Autodesk Inventor part; units mm, degrees
ref_plane "YZ Plane" through (0, 0, 0) normal (1, 0, 0) x (0, 1, 0)
ref_plane "XZ Plane" through (0, 0, 0) normal (0, 1, 0) x (-1, 0, 0)
ref_plane "XY Plane" through (0, 0, 0) normal (0, 0, 1) x (1, 0, 0)
sketch "Skizze1" plane through (0, 0, 0) normal (1, 0, 0) x (0, 1, 0)
  arc A0 (10, 59.1608) -> (10, -59.1608) centre (0, 0) ccw
  line L0 (10, 59.1608) -> (10, -9.1608)
  line L1 (10, -59.1608) -> (10, -49.1608)
  line L2 (10, -9.1608) -> (0, -9.1608)
  line L3 (0, -9.1608) -> (0, -49.1608)
  line L4 (0, -49.1608) -> (10, -49.1608)
  circle A1 centre (0, 55) radius 3
  circle A2 centre (-32.3282, 44.4959) radius 3
  circle A3 centre (-52.3081, 16.9959) radius 3
  circle A4 centre (-52.3081, -16.9959) radius 3
  circle A5 centre (-32.3282, -44.4959) radius 3
  circle A6 centre (0, -55) radius 3
  circle A7 centre (0, 0) radius 1.25
  line L5 (-7, 0) -> (-49.1993, 12.5)
  line L6 (-49.1993, 12.5) -> (-49.1993, -12.5)
  line L7 (-49.1993, -12.5) -> (-7, 0)
  line L8 (-74, 0) -> (24, 0)
  line L9 (-33.132, -38.459) -> (-5.7341, -4.015)
  line L10 (-5.7341, -4.015) -> (-47.4714, -17.9802)
  line L11 (-47.4714, -17.9802) -> (-33.132, -38.459)
  line L12 (-5.081, -50.5075) -> (-2.3941, -6.5778)
  line L13 (-2.3941, -6.5778) -> (-28.5733, -41.957)
  line L14 (-28.5733, -41.957) -> (-5.081, -50.5075)
  line L15 (-33.132, 38.459) -> (-5.7341, 4.015)
  line L16 (-5.7341, 4.015) -> (-47.4714, 17.9802)
  line L17 (-47.4714, 17.9802) -> (-33.132, 38.459)
  line L18 (-5.081, 50.5075) -> (-2.3941, 6.5778)
  line L19 (-2.3941, 6.5778) -> (-28.5733, 41.957)
  line L20 (-28.5733, 41.957) -> (-5.081, 50.5075)
  dimension "d0" = 120
  dimension "d1" = 40
  dimension "d2" = 10
  dimension "d3" = 10
  dimension "d4" = 10
  dimension "d5" = 10
  dimension "d6" = 55
  dimension "d7" = 0
  dimension "d8" = 6
  dimension "d11" = 180
  dimension "d13" = 2.5
  dimension "d19" = 33
  dimension "d20" = 12.5
  dimension "d22" = 0
  dimension "d23" = 7
  dimension "d26" = 70
  dimension "d34" = 25
extrude "Extrusion1" add sketch "Skizze1" along normal blind 10 contours L0 L8 A7 L5 L6 A0 | L8 L6 L7 A7 L0 L2 L3 L4 L1 A0
fillet "Rundung1" radius 2 15 edges at (5, -5.081, -50.5075) (5, -28.5733, -41.957) (5, -33.132, -38.459) (5, -47.4714, -17.9802) (5, -49.1993, -12.5) (5, -49.1993, 12.5) (5, -33.132, 38.459) (5, -47.4714, 17.9802) (5, -28.5733, 41.957) (5, -5.081, 50.5075) (5, -2.3941, 6.5778) (5, -5.7341, 4.015) (5, -7, 0) (5, -5.7341, -4.015) (5, -2.3941, -6.5778)
fillet "Rundung2" radius 2 4 edges at (5, 10, -9.1608) (5, 0, -9.1608) (5, 0, -49.1608) (5, 10, -49.1608)
sketch "Skizze2" plane through (10, 0, 0) normal (1, 0, 0) x (0, 0, -1)
  circle A0 centre (-16, 0) radius 0.75
  point P0 (0, 0)
  dimension "d30" = 1.5
  dimension "d31" = 16
extrude "Extrusion2" cut sketch "Skizze2" against normal blind 10
sketch "Skizze3" plane through (0, 2, -49.1608) normal (0, 0, 1) x (1, 0, 0)
  circle A0 centre (7.5, 3) radius 1.25
  line L0 (10, 6) -> (10, 0)
  line L1 (0, 6) -> (10, 6)
  point P0 (0, -2)
  dimension "d35" = 2.5
  dimension "d36" = 2.5
  dimension "d37" = 3
extrude "Extrusion3" cut sketch "Skizze3" against normal blind 12
sketch "Skizze4" plane through (0, 10, 59.1608) normal (0, 1, 0) x (1, 0, 0)
  circle A0 centre (2.5, 6) radius 1.25
  line L0 (0, 66.3216) -> (0, 0)
  line L1 (0, 0) -> (10, 0)
  point P0 (0, 59.1608)
  dimension "d40" = 2.5
  dimension "d41" = 2.5
  dimension "d42" = 6
extrude "Extrusion4" cut sketch "Skizze4" against normal blind 10
equation "\"d20\" = 0.5 * d34"
properties part number "Capstondisc"
CAD build for the part. Positions are in the model's coordinates, mm. A direction names the side the tool comes from. Give positions to 0.01 mm unless a question says otherwise; leave off trailing zeros. Order: outer loops, then holes, each group sorted by start corner. A loop starts at its lowest first (then second) coordinate and runs counter-clockwise, first axis right, second up. Notation, with made-up numbers: M 32.5,49.25 L 60.5,49.25 A15 ccw 60.5,75.25 Z; hole C 51,41 d9. An arc over 180 degrees is marked long. Put each result on its own line as item: value. Start each with the question number.
(1) Saw through at C-C, the plane z = -26.5. Write the cut outline in (x, y), then the cut area to 3 significant figures.
(2) Saw through at A-A, the plane y = 5. Write the cut outline in (x, z), then the cut area to 3 significant figures.
(3) Drill centre lines: line 1 along Y through (x, z) = (3.5, 18.5); line 2 along X through (y, z) = (5, -55); line 3 along Z through (x, y) = (5.25, -45). Where is each one in solid material? Low to high.
(4) Which spindle directions (+Z, -Z, +X, -X, +Y, -Y) get a long thin tool onto all of the face, cutting with end or side? Do faces 4 (the flat face through (5, 5, -9.161)), 5 (the cylindrical face through (5.07, -48.375, 11.44)), 6 (the flat face through (10, -10, 1)). Say none if no direction does.
(5) Saw through at B-B, the plane z = -55. Write the cut outline in (x, y).
(6) Flat gauge pins, fed straight in: pin 1 Ø4 at (x, z) = (3.5, 44.5) entering from -Y; pin 2 Ø1 at (x, y) = (4, -37.5) entering from +Z; pin 3 Ø9.5 at (y, z) = (-32.33, -44.5) entering from -X; pin 4 Ø2 at (x, y) = (6.5, -50.5) entering from +Z. Where does each tip first touch, or does it go through?
(7) Mould opens along Y. For faces 1 (the cylindrical face through (4.9, -2.4, 56.8)), 2 (the flat face through (5, 5, -49.161)), 3 (the flat face through (4.93, -20.85, -23.02)) say: +Y half, -Y half, draft (parallel to the pull), parting line (faces both ways), or undercut.
(8) Saw through at D-D, the plane z = 3.5. Write the cut outline in (x, y).
Check result:
1. outline: M 0,-53.83 L 10,-53.83 L 10,-41.51 L 0,-41.51 Z; M 0,-23.62 L 10,-23.62 L 10,-17.14 L 0,-17.14 Z; M 0,-3.61 L 10,-3.61 L 10,0 L 0,0 Z
1. area: 224 mm2
2. outline: M 0,-59.79 L 6.25,-59.79 L 6.25,-49.16 L 0,-49.16 Z; M 0,-9.16 L 10,-9.16 L 10,59.79 L 0,59.79 Z; M 8.75,-59.79 L 10,-59.79 L 10,-49.16 L 8.75,-49.16 Z; hole C 2.5,53.16 d2.5
2. area: 764 mm2
3. line 1: y = -57.08 to -54.9, -49.71 to -46.23, -17.26 to -11.22, -3.12 to 10
3. line 2: x = 0 to 6.25, 8.75 to 10
3. line 3: z = -39.69 to -21.51, -17.15 to -11.26, 11.26 to 17.15, 21.51 to 39.69
4. face 4: +X, -X, +Y
4. face 5: +X, -X
4. face 6: +Z, -Z, +X, +Y, -Y
5. outline: M 0,-23.98 L 10,-23.98 L 10,-3 L 0,-3 Z; M 0,3 L 10,3 L 10,10 L 0,10 Z; hole C 7.5,5 d2.5
6. pin 1: stops at y = -42.35
6. pin 2: stops at z = 47.23
6. pin 3: stops at x = 0
6. pin 4: stops at z = 33.91
7. face 1: undercut
7. face 2: draft
7. face 3: undercut
8. outline: M 0,-59.9 L 10,-59.9 L 10,-49.2 L 0,-49.2 Z; M 0,-18.82 L 10,-18.82 L 10,10 L 0,10 Z
